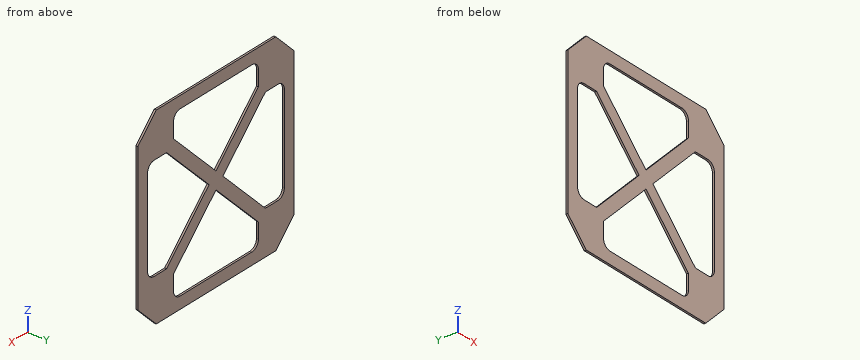
```python
from build123d import *

# Parameters (mm, degrees)
BOSS_EXTRUDE1_DEPTH = 3.175


with BuildPart() as part:
    # Sketch2 → Boss-Extrude1 (new body)
    with BuildSketch(Plane(origin=(0, 0, 0), x_dir=(1, 0, 0), z_dir=(0, 1, 0))):
        Polygon((-152.4, 116.478975516), (-116.478975516, 152.4), (116.478975516, 152.4), (152.4, 116.478975516), (152.4, -116.478975516), (116.478975516, -152.4), (-116.478975516, -152.4), (-152.4, -116.478975516), align=None)
        with BuildLine():
            Line((-82.803015062, 96.273399243), (0, 13.470384182))
            Line((0, 13.470384182), (82.803015062, 96.273399243))
            Line((82.803015062, 96.273399243), (82.803015062, 120.65))
            ThreePointArc((82.803015062, 120.65), (79.083271183, 129.630256121), (70.103015062, 133.35))
            Line((70.103015062, 133.35), (-70.103015062, 133.35))
            ThreePointArc((-70.103015062, 133.35), (-79.083271183, 129.630256121), (-82.803015062, 120.65))
            Line((-82.803015062, 120.65), (-82.803015062, 96.273399243))
        make_face(mode=Mode.SUBTRACT)
        with BuildLine():
            Line((-133.35, 70.103015062), (-133.35, -70.103015062))
            ThreePointArc((-133.35, -70.103015062), (-129.630256121, -79.083271183), (-120.65, -82.803015062))
            Line((-120.65, -82.803015062), (-96.273399243, -82.803015062))
            Line((-96.273399243, -82.803015062), (-13.470384182, 0))
            Line((-13.470384182, 0), (-96.273399243, 82.803015062))
            Line((-96.273399243, 82.803015062), (-120.65, 82.803015062))
            ThreePointArc((-120.65, 82.803015062), (-129.630256121, 79.083271183), (-133.35, 70.103015062))
        make_face(mode=Mode.SUBTRACT)
        with BuildLine():
            Line((96.273399243, 82.803015062), (120.65, 82.803015062))
            ThreePointArc((120.65, 82.803015062), (129.630256121, 79.083271183), (133.35, 70.103015062))
            Line((133.35, 70.103015062), (133.35, -70.103015062))
            ThreePointArc((133.35, -70.103015062), (129.630256121, -79.083271183), (120.65, -82.803015062))
            Line((120.65, -82.803015062), (96.273399243, -82.803015062))
            Line((96.273399243, -82.803015062), (13.470384182, 0))
            Line((13.470384182, 0), (96.273399243, 82.803015062))
        make_face(mode=Mode.SUBTRACT)
        with BuildLine():
            Line((-70.103015062, -133.35), (70.103015062, -133.35))
            ThreePointArc((70.103015062, -133.35), (79.083271183, -129.630256121), (82.803015062, -120.65))
            Line((82.803015062, -120.65), (82.803015062, -96.273399243))
            Line((82.803015062, -96.273399243), (0, -13.470384182))
            Line((0, -13.470384182), (-82.803015062, -96.273399243))
            Line((-82.803015062, -96.273399243), (-82.803015062, -120.65))
            ThreePointArc((-82.803015062, -120.65), (-79.083271183, -129.630256121), (-70.103015062, -133.35))
        make_face(mode=Mode.SUBTRACT)
    extrude(amount=BOSS_EXTRUDE1_DEPTH)


solid = part.part
```
Input: part model. Units: mm. Frame: model coordinates. Give positions to 0.01 mm unless a question says otherwise; leave off trailing zeros. Order: outer loops, then holes, each group sorted by start corner. A loop starts at its lowest first (then second) coordinate and runs counter-clockwise, first axis right, second up.
1. Material intervals for L1, parallel to Z at x = -60, y = 1.85; L2, parallel to Z at x = -14, y = 0.3; L3, parallel to X at y = 0.25, z = -45.5, sorted ascending.
Derived:
L1: z = -152.4 to -133.35, -73.47 to -46.53, 46.53 to 73.47, 133.35 to 152.4
L2: z = -152.4 to -133.35, -27.47 to -0.53, 0.53 to 27.47, 133.35 to 152.4
L3: x = -152.4 to -133.35, -58.97 to -32.03, 32.03 to 58.97, 133.35 to 152.4
2. Section C-C on x = -10. Return the cut outline in (y, z) (3 decimals).
Derived:
outline: (0, -152.4) - (3.175, -152.4) - (3.175, -133.35) - (0, -133.35) - close; (0, -23.47) - (3.175, -23.47) - (3.175, 23.47) - (0, 23.47) - close; (0, 133.35) - (3.175, 133.35) - (3.175, 152.4) - (0, 152.4) - close
3. Section B-B on z = -126.5. Return the cut outline in (x, y) (3 decimals), and give its area (3 significant figures).
Derived:
outline: (-142.379, 0) - (-81.375, 0) - (-81.375, 3.175) - (-142.379, 3.175) - close; (81.375, 0) - (142.379, 0) - (142.379, 3.175) - (81.375, 3.175) - close
area: 387 mm2
4. Section A-A on x = -102. Return the cut outline in (y, z) (3 decimals).
Derived:
outline: (0, -152.4) - (3.175, -152.4) - (3.175, -82.803) - (0, -82.803) - close; (0, 82.803) - (3.175, 82.803) - (3.175, 152.4) - (0, 152.4) - close
5. Section D-D on z = 53. Return the cut outline in (x, y) (3 decimals), and give its area (3 significant figures).
Derived:
outline: (-152.4, 0) - (-133.35, 0) - (-133.35, 3.175) - (-152.4, 3.175) - close; (-66.47, 0) - (-39.53, 0) - (-39.53, 3.175) - (-66.47, 3.175) - close; (39.53, 0) - (66.47, 0) - (66.47, 3.175) - (39.53, 3.175) - close; (133.35, 0) - (152.4, 0) - (152.4, 3.175) - (133.35, 3.175) - close
area: 292 mm2
